Input: part model. Units: mm. Frame: model coordinates. Face numbers are marked on the shaded views. A direction names the side the tool comes from. Coordinates: 2 decimals unless noted, no trailing zeros. Loops run counter-clockwise (first coordinate to the right, second up) from the corner with the lowest first, then second, coordinate; pieces in that order, holes last. Notation, with made-up numbers: M 36,-21 L 53,-21 A21 cw 53,-14 Z; hole C 28.5,-14.75 d9. An arc over 180 degrees is marked long. Use a Markdown table: item, result. Add a question column.
1. Section C-C on x = -23. Output: boundary loops of the cut face in (y, z), then the cut area to 3 significant figures.
2. Set-up query: the marked faces 4, 5 and 6. Return all of +Z, -Z, +X, -X, +Y, -Y with unobstructed straight access to the full face (end or side cutting, diameter ignored); none if empty.
3. Line query: L1, parallel to X at y = 22.5, z = 21; L2, parallel to X at y = 21.5, z = 7.75; L3, parallel to Z at x = 19.5, y = 28. Output: solid intervals per line, ascending. Write a range as [from, to].
4. Pin query (flat end, axial travel): pin 1 (5 mm diameter, centred on x = 9, z = 7.5, fed in from -Y); pin 2 (23 mm diameter, centred on x = 9.94, y = 14.4, fed in from +Z); pin 3 (6 mm diameter, centred on y = -18.5, z = 8, fed in from -X); pin 4 (10 mm diameter, centred on x = 8.5, y = 9, fed in from -Z). Return the tip coordinate at first contact, or that it passes through.
5. Section B-B on y = 16. State how many separate pieces and enclosed holes the cut face has, then the cut area to 3 significant figures.
6. Draft query along Y for the marked faces 1, 2 and 3. Return one class per face: +Y half, -Y half, draft (parallel to the pull), parting line (faces both ways), or undercut.
7. Section D-D on x = 25. Output: boundary loops of the cut face in (y, z), then the cut area to 3 significant figures.
8. Section A-A on z = 16.5. Output: boundary loops of the cut face in (x, y), then the cut area to 3 significant figures.
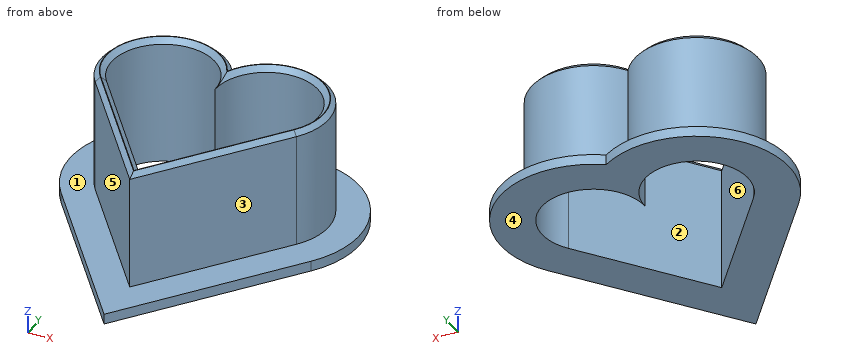
```python
from build123d import *

# Parameters (mm, degrees)
F1_DEPTH = 25
F2_SIZE  = 1
F3_SIZE  = 0.9
F4_DEPTH = 2


with BuildPart() as f1:
    # F0 (on Top) → F1 (new body)
    with BuildSketch(Plane.XY):
        with BuildLine():
            ThreePointArc((19.4576948641, 7.0878110017), (16.9014285769, 24.177453273), (-0.0826562467, 20.994493487))
            ThreePointArc((-0.0826562467, 20.994493487), (-17.0758205861, 24.0547884178), (-19.5363304351, 6.9644715509))
            Line((-19.5363304351, 6.9644715509), (0.0076825592, -18.2174257356))
            Line((0.0076825592, -18.2174257356), (19.4576948641, 7.0878110017))
        make_face()
        with BuildLine():
            Line((17.8719759612, 8.3066200764), (0, -14.9455288462))
            Line((0, -14.9455288462), (-17.9563526213, 8.1907138222))
            ThreePointArc((-17.9563526213, 8.1907138222), (-13.3155361336, 23.7759426267), (-0.056541053, 14.3612953145))
            ThreePointArc((-0.056541053, 14.3612953145), (13.1429709457, 23.8749795171), (17.8719759612, 8.3066200764))
        make_face(mode=Mode.SUBTRACT)
    extrude(amount=F1_DEPTH)

    # F2
    f2_edges = [f1.edges().sort_by_distance(p)[0] for p in [
        (-8.978176, -3.377408, 25),
        (8.935988, -3.319454, 25),
        (13.142971, 23.87498, 25),
        (-13.315536, 23.775943, 25),
    ]]
    chamfer(f2_edges, length=F2_SIZE)

    # F3
    f3_edges = [f1.edges().sort_by_distance(p)[0] for p in [
        (-9.764324, -5.626477, 25),
        (-17.075821, 24.054788, 25),
        (16.901429, 24.177453, 25),
        (9.732689, -5.564807, 25),
    ]]
    chamfer(f3_edges, length=F3_SIZE)

    # F0 (on Top) → F4 (join)
    with BuildSketch(Plane.XY):
        with BuildLine():
            Line((0.0307302369, -28.033116404), (24.214851573, 3.4313837773))
            ThreePointArc((24.214851573, 3.4313837773), (23.0617943824, 26.7257310501), (-0.1154648769, 29.3278088692))
            ThreePointArc((-0.1154648769, 29.3278088692), (-23.2520807017, 26.5642978264), (-24.2762638766, 3.285744737))
            Line((-24.2762638766, 3.285744737), (0.0307302369, -28.033116404))
        make_face()
        with BuildLine():
            ThreePointArc((-19.5363304351, 6.9644715509), (-17.0758205861, 24.0547884178), (-0.0826562467, 20.994493487))
            ThreePointArc((-0.0826562467, 20.994493487), (16.9014285769, 24.177453273), (19.4576948641, 7.0878110017))
            Line((19.4576948641, 7.0878110017), (0.0076825592, -18.2174257356))
            Line((0.0076825592, -18.2174257356), (-19.5363304351, 6.9644715509))
        make_face(mode=Mode.SUBTRACT)
    extrude(amount=F4_DEPTH)


solid = f1.part
```
Answers below:
| question | item | result |
|---|---|---|
| 1 | outline | M 1.64,0 L 26.83,0 L 26.83,2 L 1.64,2 Z |
| 1 | area | 50.4 mm² |
| 2 | face 4 | -Z, +X, -X, +Y, -Y |
| 2 | face 5 | +Z, -X, -Y |
| 2 | face 6 | +Z, -Z |
| 3 | L1 | x = [-18.84, -15.81], [-4.3, -1.27], [1.09, 4.08], [15.81, 18.8] |
| 3 | L2 | x = [-19.67, -17.02], [-3.09, -0.44], [0.27, 2.9], [16.99, 19.62] |
| 3 | L3 | z = [0, 2] |
| 4 | pin 1 | stops at y = -9.77 |
| 4 | pin 2 | stops at z = 25 |
| 4 | pin 3 | stops at x = -2.1 |
| 4 | pin 4 | passes through |
| 5 | separate pieces | 3 |
| 5 | enclosed holes | 0 |
| 5 | area | 130 mm² |
| 6 | face 1 | draft |
| 6 | face 2 | undercut |
| 6 | face 3 | -Y half |
| 7 | outline | M 4.54,0 L 24.26,0 L 24.26,2 L 4.54,2 Z |
| 7 | area | 39.5 mm² |
| 8 | outline | M -19.54,6.96 L 0.01,-18.22 L 19.46,7.09 A12 ccw long -0.08,20.99 A12 ccw long Z; hole M -17.96,8.19 L 0,-14.95 L 17.87,8.31 A10 ccw long -0.06,14.36 A10 ccw long Z |
| 8 | area | 272 mm² |
